Geometry check sheet. Reference: the model listing, model coordinates, mm. Face numbers are marked on the shaded views. Give positions to 0.01 mm unless a question says otherwise; leave off trailing zeros. Loops run counter-clockwise (first coordinate to the right, second up) from the corner with the lowest first, then second, coordinate; pieces in that order, holes last. Notation, with made-up numbers: (45, 34.25) -> (73, 34.25) arc R31 cw to (73, 58.25) -> close; hole circle Ø2 at (26.25, -32). An arc over 180 degrees is marked (long way). One line per question, with ' | ' between items.
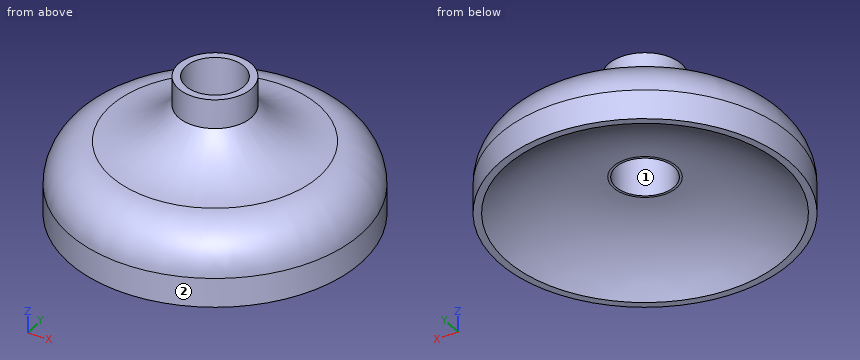
from build123d import *

# Parameters (mm, degrees)
SKETCH1_R           = 100
SKETCH1_R_2         = 95
BOSS_EXTRUDE1_DEPTH = 25
SKETCH2_R           = 100
BOSS_EXTRUDE2_DEPTH = 25
SKETCH3_R           = 20
CUT_EXTRUDE1_DEPTH  = 25
BOSS_EXTRUDE3_START = 25
SKETCH4_R           = 25
SKETCH4_R_2         = 20
BOSS_EXTRUDE3_DEPTH = 25
FILLET1_R           = 30
FILLET2_R           = 120
FILLET3_R           = 60
BOSS_EXTRUDE4_START = 20
SKETCH5_R           = 25
SKETCH5_R_2         = 20
BOSS_EXTRUDE4_DEPTH = 20


with BuildPart() as part:
    # Sketch1 → Boss-Extrude1 (new body)
    with BuildSketch(Plane.XY):
        Circle(SKETCH1_R)
        Circle(SKETCH1_R_2, mode=Mode.SUBTRACT)
    extrude(amount=BOSS_EXTRUDE1_DEPTH)

    # Sketch2 → Boss-Extrude2 (add)
    with BuildSketch(Plane.XY.offset(25)):
        Circle(SKETCH2_R)
    extrude(amount=BOSS_EXTRUDE2_DEPTH)

    # Sketch3 → Cut-Extrude1 (cut)
    with BuildSketch(Plane.XY.offset(50)):
        Circle(SKETCH3_R)
    extrude(amount=-CUT_EXTRUDE1_DEPTH, mode=Mode.SUBTRACT)

    # Sketch4 → Boss-Extrude3 (add)
    with BuildSketch(Plane.XY.offset(50).offset(BOSS_EXTRUDE3_START)):
        Circle(SKETCH4_R)
        Circle(SKETCH4_R_2, mode=Mode.SUBTRACT)
    extrude(amount=-BOSS_EXTRUDE3_DEPTH)

    # Fillet1
    fillet1_edges = [part.edges().sort_by_distance(p)[0] for p in [
        (-100, 0, 50),
    ]]
    fillet(fillet1_edges, radius=FILLET1_R)

    # Fillet2
    # the kernel refuses this fillet: 120 mm, written as the material it adds along each edge
    with BuildSketch(Plane(origin=(0, 0, 25), x_dir=(1, 0, 0), z_dir=(0, -1, 0))) as fillet2_piece_1:
        with BuildLine():
            CenterArc((21.685608507, -120), FILLET2_R, 52.341537994, 37.658462006)
            Line((21.685608507, 0), (21.685608507, 2.4))
            Line((21.685608507, 2.4), (95, 2.4))
            Line((95, 2.4), (97.4, 0))
            ThreePointArc((97.4, 0), (97.4, -12.5), (96.46628783, -23.1))
            Line((96.46628783, -23.1), (95, -25))
        make_face()
    revolve(axis=Axis((0, 0, 25), (0, 0, 1)))

    # Fillet3
    # the kernel refuses this fillet: 60 mm, written as the material it adds along each edge
    with BuildSketch(Plane(origin=(0, 0, 50), x_dir=(1, 0, 0), z_dir=(0, -1, 0))) as fillet3_piece_1_section:
        with BuildLine():
            CenterArc((73.791247331, 59.920111453), FILLET3_R, 215.59146616, 51.994236434)
            Line((71.26374911, -0.026629516), (71.010999288, -6.021303613))
            ThreePointArc((71.010999288, -6.021303613), (70, -6), (25, -6))
            Line((25, -6), (19, 0))
            ThreePointArc((19, 0), (19, 12.5), (20.120875267, 21.507988855))
            Line((20.120875267, 21.507988855), (25, 25))
        make_face()
    fillet3_piece_1 = revolve(axis=Axis((0, 0, 50), (0, 0, 1)), mode=Mode.PRIVATE)
    fillet3_piece_1 = fillet3_piece_1 - Plane(origin=(0, 0, 57.041337481), x_dir=(1, 0, 0), z_dir=(0, 0, 1)) * Cylinder(20, 286, mode=Mode.PRIVATE)
    add(fillet3_piece_1)

    # Sketch5 → Boss-Extrude4 (add)
    with BuildSketch(Plane.XY.offset(75).offset(BOSS_EXTRUDE4_START)):
        Circle(SKETCH5_R)
        Circle(SKETCH5_R_2, mode=Mode.SUBTRACT)
    extrude(amount=-BOSS_EXTRUDE4_DEPTH)


solid = part.part
Item 1: Depth check by flat-ended pin: pin 1 Ø6 at (x, y) = (11.5, 20) entering from -Z; pin 2 Ø3 at (x, z) = (-50, 27) entering from +Y; pin 3 Ø8 at (x, z) = (-26.5, 21) entering from -Y. Enter the tip coordinate at first touch or a pass-through.
Result:
pin 1: z = 24.92 | pin 2: y = 86.59 | pin 3: y = -97.43
Item 2: Sectioned sample at A-A (z = 85). Record the cut outline in (x, y), plus the area to 3 significant figures.
Result:
outline: circle Ø50 at (0, 0); hole circle Ø40 at (0, 0) | area: 707 mm2
Item 3: Release check for a two-part mould opening along Y. For the marked faces 1 and 2 record: pulls with the +Y half, pulls with the -Y half, needs draft (parallel to the pull), parting line crosses it, or undercut.
Result:
face 1: undercut | face 2: parting line crosses it
Item 4: Scan lines: probe 1 along Y at (x, z) = (-6, 66.5); probe 2 along Y at (x, z) = (-6, 85.5); probe 3 along Z at (x, y) = (37, -90.5). Record each from-to range of solid material in increasing order.
Result:
probe 1: -31.82 to -19.08, 19.08 to 31.82 | probe 2: -24.27 to -19.08, 19.08 to 24.27 | probe 3: 0 to 31.35
